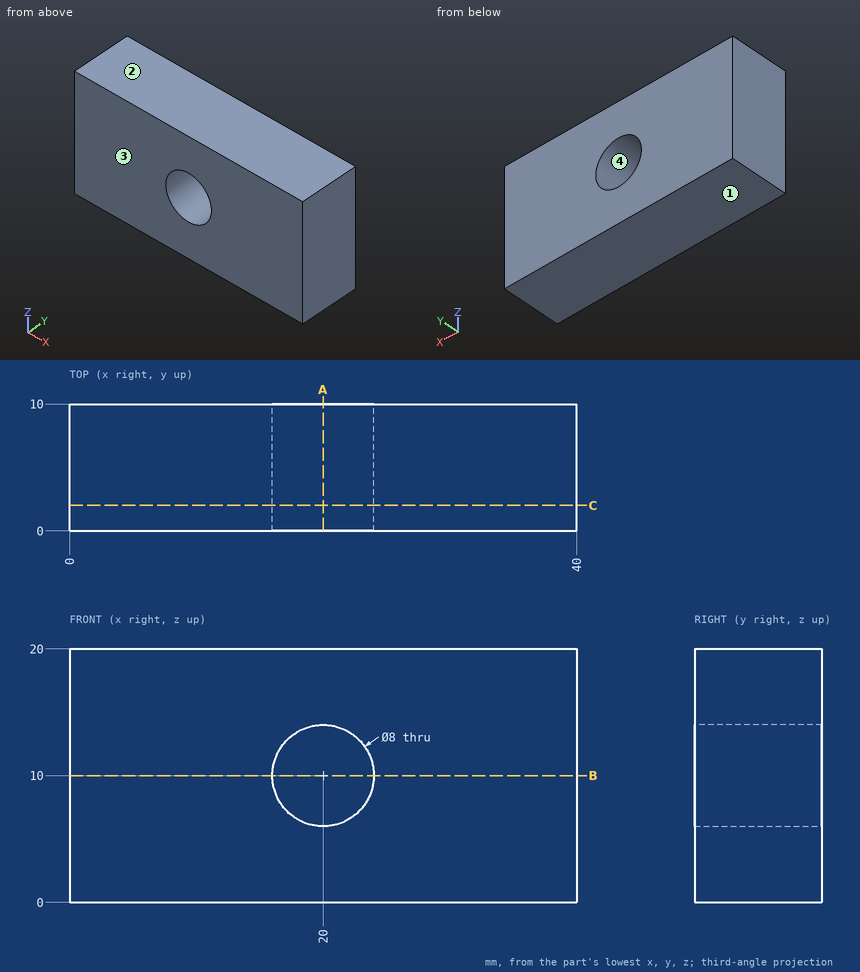
The drawing under review shows one solid part. Ordinate dimensions are in mm from its lowest x, y, z. Give positions to 0.01 mm unless a question says otherwise; leave off trailing zeros. Write each loop counter-clockwise with the first axis right and the second up, starting at its lowest first coordinate (ties: lowest second). Pieces come first, ordered by that corner, then holes. Notation, with made-up numbers: M 55.25,8 L 73.25,8 A26 ccw 73.25,44 Z; hole C 15,83 d3. An arc over 180 degrees is marked long. Write each question's results on one line, items separated by ' | '. Start each with the question number.
1. We need section B-B (z = 10). Write out the cut boundary in (x, y), and give its area (3 significant figures).
2. We need section A-A (x = 20). Write out the cut boundary in (y, z), and give its area (3 significant figures).
3. We need section C-C (y = 2). Write out the cut boundary in (x, z).
4. Mouldability with a two-part tool opening along Z and no side actions: class the marked faces 1, 2, 3 and 4 as released by +Z, released by -Z, zero draft, split by the parting line, or undercut.
5. For probe 1 along X at (y, z) = (2.25, 10); probe 2 along Z at (x, y) = (19.5, 8.75); probe 3 along Z at (x, y) = (17, 8), list the stretches that pass through material, from the lowest coordinate up. Write a range as [from, to].
Results found:
1) outline: M 0,0 L 16,0 L 16,10 L 0,10 Z; M 24,0 L 40,0 L 40,10 L 24,10 Z | area: 320 mm^2
2) outline: M 0,0 L 10,0 L 10,6 L 0,6 Z; M 0,14 L 10,14 L 10,20 L 0,20 Z | area: 120 mm^2
3) outline: M 0,0 L 40,0 L 40,20 L 0,20 Z; hole C 20,10 d8
4) face 1: released by -Z | face 2: released by +Z | face 3: zero draft | face 4: undercut
5) probe 1: x = [0, 16], [24, 40] | probe 2: z = [0, 6.03], [13.97, 20] | probe 3: z = [0, 7.35], [12.65, 20]
